For this review, take the finished solid that the model builds, in its own axes (mm). Face numbers are marked on the shaded views. A direction names the side the tool comes from. Round coordinates to 2 decimals unless told otherwise and drop trailing zeros. Order: outer loops, then holes, each group sorted by start corner. A loop starts at its lowest first (then second) coordinate and runs counter-clockwise, first axis right, second up. Notation, with made-up numbers: (-17, 81) -> (30, 81) arc R30 ccw to (30, 116) -> close; hole circle Ø1 at (17, -21.75). An arc over 180 degrees is marked (long way). Answer in a Markdown table with one row per item.
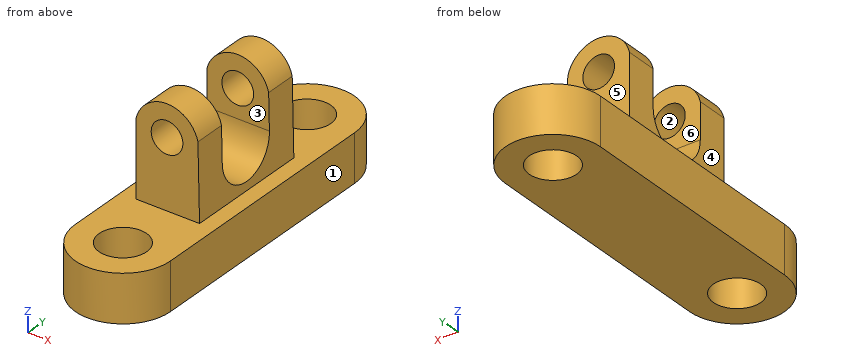
```python
from build123d import *

# Parameters (mm, degrees)
F0_W      = 38.1
F0_H      = 99.228098
F1_DEPTH  = 19.05
F2_R      = 9.525
F3_DEPTH  = 127
F5_DEPTH  = 25.4
F6_R      = 6.35
F7_DEPTH  = 127
F9_DEPTH  = 63.5
F10_DEPTH = 127


with BuildPart() as f1:
    # F0 (on Top) → F1 (new body)
    with BuildSketch(Plane.XY):
        Rectangle(F0_W, F0_H)
        with BuildLine():
            Line((-19.05, 49.614049), (19.05, 49.614049))
            ThreePointArc((19.05, 49.614049), (0, 68.664049), (-19.05, 49.614049))
        make_face()
        with BuildLine():
            ThreePointArc((-19.05, -49.614049), (0, -68.664049), (19.05, -49.614049))
            Line((19.05, -49.614049), (-19.05, -49.614049))
        make_face()
    extrude(amount=F1_DEPTH)

    # F2 (on face) → F3 (cut)
    with BuildSketch(Plane.XY.offset(19.05)):
        with Locations((0, 49.614049)):
            Circle(F2_R)
        with Locations((0, -49.614049)):
            Circle(F2_R)
    extrude(amount=-F3_DEPTH, mode=Mode.SUBTRACT)

    # F4 (on Front) → F5 (join, symmetric)
    with BuildSketch(Plane.XZ):
        with BuildLine():
            Line((-12.7, 19.05), (0, 19.05))
            Line((0, 19.05), (12.7, 19.05))
            Line((12.7, 19.05), (12.045477, 49.522972))
            ThreePointArc((12.045477, 49.522972), (-0.324468, 59.36199), (-12.7, 49.53))
            Line((-12.7, 49.53), (-12.7, 19.05))
        make_face()
    extrude(amount=F5_DEPTH, both=True)

    # F6 (on face) → F7 (cut)
    with BuildSketch(Plane(origin=(0, 25.4, 0), x_dir=(-1, 0, 0), z_dir=(0, 1, 0))):
        with Locations((0.328075, 46.661991)):
            Circle(F6_R)
    extrude(amount=-F7_DEPTH, mode=Mode.SUBTRACT)

    # F8 (on Right) → F9 (cut, symmetric)
    with BuildSketch(Plane.YZ):
        with BuildLine():
            Line((12.7, 35.172723), (12.7, 75.489088))
            Line((12.7, 75.489088), (-12.7, 75.489088))
            Line((-12.7, 75.489088), (-12.7, 35.172723))
            ThreePointArc((-12.7, 35.172723), (0, 22.472723), (12.7, 35.172723))
        make_face()
    extrude(amount=F9_DEPTH, both=True, mode=Mode.SUBTRACT)

    # F8 (on Right) → F10 (cut, symmetric)
    with BuildSketch(Plane.YZ):
        with BuildLine():
            Line((12.7, 35.172723), (12.7, 75.489088))
            Line((12.7, 75.489088), (-12.7, 75.489088))
            Line((-12.7, 75.489088), (-12.7, 35.172723))
            ThreePointArc((-12.7, 35.172723), (0, 22.472723), (12.7, 35.172723))
        make_face()
    extrude(amount=F10_DEPTH, both=True, mode=Mode.SUBTRACT)


solid = f1.part
```
Q1. Tool access review of the marked faces 4, 5 and 6: name each direction out of +Z, -Z, +X, -X, +Y, -Y from which nothing blocks a thin tool from reaching the whole face with its end or side.
Answer key:
| item | result |
|---|---|
| face 4 | +Z, -X, +Y, -Y |
| face 5 | +Z, +X, -X, +Y |
| face 6 | +Z, +X, -X |
Q2. Take a section at B-B, the plane z = 9.5. Write out the cut boundary in (x, y) (3 decimals), then the cut area to 3 significant figures.
Answer key:
| item | result |
|---|---|
| outline | (-19.05, -49.614) arc R19.05 ccw to (19.05, -49.614) -> (19.05, 49.614) arc R19.05 ccw to (-19.05, 49.614) -> close; hole circle Ø19.05 at (0, -49.614); hole circle Ø19.05 at (0, 49.614) |
| area | 4,350 mm^2 |
Q3. Clearance check with flat-ended pins moving along their axes: pin 1 Ø16.5 at (x, z) = (-0.33, 46.66) entering from +Y; pin 2 Ø1.5 at (x, y) = (-14.5, 36) entering from -Z; pin 3 Ø14.5 at (x, z) = (-0.33, 46.66) entering from -Y; pin 4 Ø1.5 at (x, y) = (-2, 1.5) entering from +Z. State where each tip first meets the part, or that it passes through.
Answer key:
| item | result |
|---|---|
| pin 1 | stops at y = 25.4 |
| pin 2 | stops at z = 0 |
| pin 3 | stops at y = -25.4 |
| pin 4 | stops at z = 22.67 |
Q4. Take a section at A-A, the plane x = 0. Write out the cut boundary in (y, z).
Answer key:
| item | result |
|---|---|
| outline | (-68.66, 0) -> (-59.14, 0) -> (-59.14, 19.05) -> (-68.66, 19.05) -> close; (-40.09, 0) -> (40.09, 0) -> (40.09, 19.05) -> (25.4, 19.05) -> (25.4, 40.32) -> (12.7, 40.32) -> (12.7, 35.17) arc R12.7 cw to (-12.7, 35.17) -> (-12.7, 40.32) -> (-25.4, 40.32) -> (-25.4, 19.05) -> (-40.09, 19.05) -> close; (-25.4, 53) -> (-12.7, 53) -> (-12.7, 59.36) -> (-25.4, 59.36) -> close; (12.7, 53) -> (25.4, 53) -> (25.4, 59.36) -> (12.7, 59.36) -> close; (59.14, 0) -> (68.66, 0) -> (68.66, 19.05) -> (59.14, 19.05) -> close |
Q5. The part is to be moulded in two halves that separate along X. For the marked faces 1, 2 and 3, say which applies: +X half, -X half, draft (parallel to the pull), parting line (faces both ways), or undercut.
Answer key:
| item | result |
|---|---|
| face 1 | +X half |
| face 2 | undercut |
| face 3 | draft |
Q6. Take a section at C-C, the plane y = -45. Write out the cut boundary in (x, z).
Answer key:
| item | result |
|---|---|
| outline | (-19.05, 0) -> (-8.33, 0) -> (-8.33, 19.05) -> (-19.05, 19.05) -> close; (8.33, 0) -> (19.05, 0) -> (19.05, 19.05) -> (8.33, 19.05) -> close |
Q7. To check wall thickness, follow probe 1 along Y at (x, z) = (-10, 38); probe 2 along Y at (x, z) = (-6, 3); probe 3 along Y at (x, z) = (5.5, 13.5). State the ranges of each line that lie inside material, in increasing order.
Answer key:
| item | result |
|---|---|
| probe 1 | y = -25.4 to -12.7, 12.7 to 25.4 |
| probe 2 | y = -67.69 to -57.01, -42.22 to 42.22, 57.01 to 67.69 |
| probe 3 | y = -67.85 to -57.39, -41.84 to 41.84, 57.39 to 67.85 |
Q8. Take a section at D-D, the plane z = 26. Write out the cut boundary in (x, y), then the cut area to 3 significant figures.
Answer key:
| item | result |
|---|---|
| outline | (-12.7, -25.4) -> (12.55, -25.4) -> (12.55, -8.78) -> (-12.7, -8.78) -> close; (-12.7, 8.78) -> (12.55, 8.78) -> (12.55, 25.4) -> (-12.7, 25.4) -> close |
| area | 839 mm^2 |
